Source: CAD feature listing. Evaluate the final solid. Frame: model axes, mm. A direction names the side the tool comes from. Round coordinates to 2 decimals unless told otherwise and drop trailing zeros. Write each loop counter-clockwise with the first axis right and the second up, starting at its lowest first coordinate (ties: lowest second). Pieces come first, ordered by that corner, then holes.
```python
from build123d import *

# Parameters (mm, degrees)
SKETCH1_R           = 10.16
BOSS_EXTRUDE1_DEPTH = 12.7
CUT_EXTRUDE1_START  = 12.7
SKETCH2_R           = 14.2875
CUT_EXTRUDE1_DEPTH  = 4


with BuildPart() as part:
    # Sketch1 → Boss-Extrude1 (new body)
    with BuildSketch(Plane.XY):
        Polygon((14, -56), (-32, -56), (-32, 0), (-32, 30), (32, 30), (32, -28.77498914), (14, -28.77498914), align=None)
        Circle(SKETCH1_R, mode=Mode.SUBTRACT)
    extrude(amount=BOSS_EXTRUDE1_DEPTH)

    # Sketch2 → Cut-Extrude1 (cut)
    with BuildSketch(Plane.XY.offset(CUT_EXTRUDE1_START)):
        Circle(SKETCH2_R)
    extrude(amount=-CUT_EXTRUDE1_DEPTH, mode=Mode.SUBTRACT)


solid = part.part
```
Q1. Set-up query: faces 5 (the face through (14, -42, 6)), 6 (the face through (32, 1, 6)). Return all of +Z, -Z, +X, -X, +Y, -Y with unobstructed straight access to the full face (end or side cutting, diameter ignored); none if empty.
Q2. Pin query (flat end, axial travel): P1, Ø10, axis at x = 20.5, y = -36, coming from the -Z side; P2, Ø8.5, axis at x = 7, y = 2.5, coming from the +Z side; P3, Ø4, axis at x = 25.5, z = 5, coming from the -Y side (3 decimals); P4, Ø6.5, axis at y = -43.5, z = 3.5, coming from the +X side. Return the tip coordinate at first contact, or that it passes through.
Q3. Line query: line 1 (Y direction, x = 0, z = 6); line 2 (X direction, y = 0, z = 2.75); line 3 (Y direction, x = 0, z = 10.05). Output: solid intervals per line, ascending.
Q4. Mould query, pull axis Y, two halves, no side actions, for faces 1 (the face through (-10, -3, 8.7)), 2 (the face through (23, -28.775, 6)), 3 (the face through (7.6, -12.4, 12.7)), 4 (the face through (-14.274, 0.628, 10.728)). Classes: pulls with the +Y half, pulls with the -Y half, needs draft (parallel to the pull), parting line crosses it, or undercut.
Q5. Section query A-A, the plane y = 0. Output: boundary loops of the cut face in (x, z).
Q6. Section query B-B, the plane z = 1. Output: boundary loops of the cut face in (x, y).
Q7. Section query D-D, the plane y = -35. Output: boundary loops of the cut face in (x, z), and give its area (3 significant figures).
Q8. Section query C-C, the plane x = 23. Output: boundary loops of the cut face in (y, z).
Filled in:
1. face 5: +Z, -Z, +X, -Y
1. face 6: +Z, -Z, +X, +Y, -Y
2. P1: passes through
2. P2: stops at z = 8.7
2. P3: stops at y = -28.775
2. P4: stops at x = 14
3. line 1: y = -56 to -10.16, 10.16 to 30
3. line 2: x = -32 to -10.16, 10.16 to 32
3. line 3: y = -56 to -14.29, 14.29 to 30
4. face 1: undercut
4. face 2: pulls with the -Y half
4. face 3: needs draft
4. face 4: undercut
5. outline: (-32, 0) - (-10.16, 0) - (-10.16, 8.7) - (-14.29, 8.7) - (-14.29, 12.7) - (-32, 12.7) - close; (10.16, 0) - (32, 0) - (32, 12.7) - (14.29, 12.7) - (14.29, 8.7) - (10.16, 8.7) - close
6. outline: (-32, -56) - (14, -56) - (14, -28.77) - (32, -28.77) - (32, 30) - (-32, 30) - close; hole circle Ø20.32 at (0, 0)
7. outline: (-32, 0) - (14, 0) - (14, 12.7) - (-32, 12.7) - close
7. area: 584 mm2
8. outline: (-28.77, 0) - (30, 0) - (30, 12.7) - (-28.77, 12.7) - close
